Geometry: see drawing. Coordinates: mm, zero at the bounding-box minimum. A direction names the side the tool comes from. Coordinates: 2 decimals unless noted, no trailing zeros. Loops run counter-clockwise (first coordinate to the right, second up) from the corner with the lowest first, then second, coordinate; pieces in that order, holes last. Notation, with made-up numbers: M 82.25,42.25 L 89.25,42.25 A7 ccw 89.25,50.25 Z; hole C -8,68.25 d8. An arc over 180 degrees is marked long. Write each question's results on one line, items separated by ' | '. Start each with the question number.
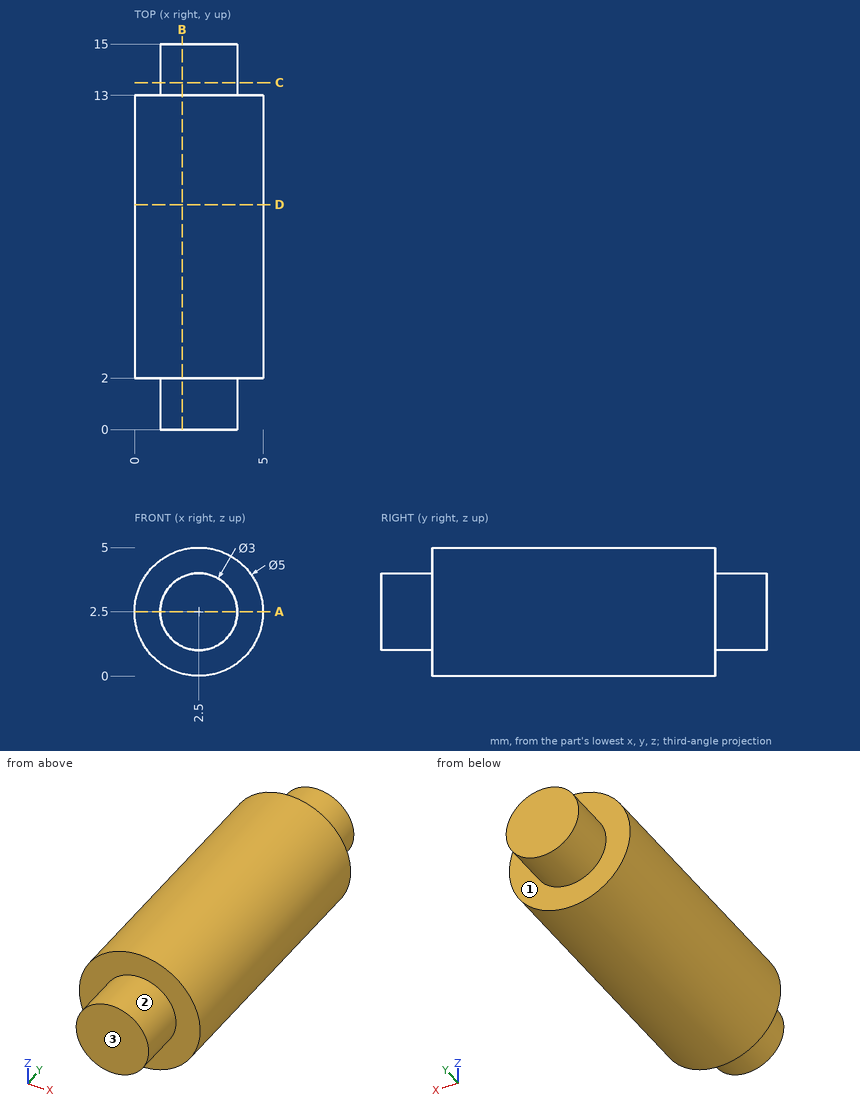
Item 1: Cut plane D-D (y = 8.75). Output: boundary loops of the cut face in (x, z), then the cut area to 3 significant figures.
Item 2: Cut plane A-A (z = 2.5). Output: boundary loops of the cut face in (x, y), then the cut area to 3 significant figures.
Item 3: Access query for the marked faces 1, 2 and 3. Directions: +Z, -Z, +X, -X, +Y, -Y. A direction counts if a zero-diameter tool reaches every point of the face in a straight line with its end or side. Return the directions, or none.
Item 4: Cut plane C-C (y = 13.5). Output: boundary loops of the cut face in (x, z), then the cut area to 3 significant figures.
Item 5: Cut plane B-B (x = 1.85). Output: boundary loops of the cut face in (y, z).
Item 6: Line query: probe 1 along Z at (x, y) = (2.6, 7); probe 2 along Y at (x, z) = (4.35, 2.5); probe 3 along Z at (x, y) = (0.65, 9.25). Output: solid intervals per line, ascending.
Response values:
1) outline: C 2.5,2.5 d5 | area: 19.6 mm2
2) outline: M 0,2 L 1,2 L 1,0 L 4,0 L 4,2 L 5,2 L 5,13 L 4,13 L 4,15 L 1,15 L 1,13 L 0,13 Z | area: 67.0 mm2
3) face 1: +Y | face 2: -Y | face 3: +Z, -Z, +X, -X, -Y
4) outline: C 2.5,2.5 d3 | area: 7.07 mm2
5) outline: M 0,1.15 L 2,1.15 L 2,0.09 L 13,0.09 L 13,1.15 L 15,1.15 L 15,3.85 L 13,3.85 L 13,4.91 L 2,4.91 L 2,3.85 L 0,3.85 Z
6) probe 1: z = 0 to 5 | probe 2: y = 2 to 13 | probe 3: z = 0.82 to 4.18
